```python
from build123d import *

# Parameters (mm, degrees)
BOSS_EXTRUDE1_START     = 7.2
SKETCH1_W               = 6
SKETCH1_H               = 3
BOSS_EXTRUDE1_DEPTH     = 24.3
BOSS_EXTRUDE2_START     = 28.5
SKETCH2_W               = 3
SKETCH2_H               = 35.475
BOSS_EXTRUDE2_DEPTH     = 21.5
CUT_EXTRUDE1_DEPTH      = 60.023009285
CUT_EXTRUDE1_DEPTH_BACK = 60.023009285
SKETCH3_R               = 1.2
SKETCH3_R_2             = 0.9
CUT_EXTRUDE2_DEPTH      = 60.023009285
CUT_EXTRUDE2_DEPTH_BACK = 60.023009285
SKETCH4_W               = 11
SKETCH4_H               = 1.2
SKETCH4_W_2             = 17
SKETCH4_H_2             = 12.475
CUT_EXTRUDE3_DEPTH      = 60.023009285
CUT_EXTRUDE3_DEPTH_BACK = 60.023009285
SKETCH5_W               = 3
SKETCH5_H               = 2.5


with BuildPart() as part:
    # Sketch1 → Boss-Extrude1 (new body)
    with BuildSketch(Plane.XY.offset(BOSS_EXTRUDE1_START)):
        with Locations((17.8, 21.975)):
            Rectangle(SKETCH1_W, SKETCH1_H)
    extrude(amount=BOSS_EXTRUDE1_DEPTH)

    # Sketch2 → Boss-Extrude2 (add)
    with BuildSketch(Plane.XY.offset(BOSS_EXTRUDE2_START)):
        with Locations((17.8, 5.7375)):
            Rectangle(SKETCH2_W, SKETCH2_H)
    extrude(amount=BOSS_EXTRUDE2_DEPTH)

    # Sketch3 → Cut-Extrude1 (cut, two sides: drawn at the far end of the back side and taken through both)
    with BuildSketch(Plane(origin=(0, 0, 0), x_dir=(1, 0, 0), z_dir=(0, 1, 0)).offset(-CUT_EXTRUDE1_DEPTH_BACK)):
        with Locations(Location((17.8, -24.5, 0), (0, 0, 270))):
            Circle(SKETCH3_R)
        with Locations(Location((17.8, -10.2, 0), (0, 0, 270))):
            Circle(SKETCH3_R_2)
    extrude(amount=CUT_EXTRUDE1_DEPTH + CUT_EXTRUDE1_DEPTH_BACK, mode=Mode.SUBTRACT)

    # Sketch4 → Cut-Extrude2 (cut, two sides: drawn at the far end of the back side and taken through both)
    with BuildSketch(Plane(origin=(0, 0, 0), x_dir=(0, 0, -1), z_dir=(1, 0, 0)).offset(-CUT_EXTRUDE2_DEPTH_BACK)):
        with Locations((-45.5, -6)):
            Rectangle(SKETCH4_W, SKETCH4_H)
        with Locations((-45.5, 0)):
            Rectangle(SKETCH4_W, SKETCH4_H)
        with Locations((-45.5, 6)):
            Rectangle(SKETCH4_W, SKETCH4_H)
        with Locations((-42.5, 18.2375)):
            Rectangle(SKETCH4_W_2, SKETCH4_H_2)
    extrude(amount=CUT_EXTRUDE2_DEPTH + CUT_EXTRUDE2_DEPTH_BACK, mode=Mode.SUBTRACT)

    # Sketch5 → Cut-Extrude3 (cut, two sides: drawn at the far end of the back side and taken through both)
    with BuildSketch(Plane(origin=(0, 0, 0), x_dir=(0, 0, -1), z_dir=(1, 0, 0)).offset(-CUT_EXTRUDE3_DEPTH_BACK)):
        with Locations((-49.5, -11.75)):
            Rectangle(SKETCH5_W, SKETCH5_H)
        with Locations((-49.5, 11.75)):
            Rectangle(SKETCH5_W, SKETCH5_H)
    extrude(amount=CUT_EXTRUDE3_DEPTH + CUT_EXTRUDE3_DEPTH_BACK, mode=Mode.SUBTRACT)


solid = part.part
```
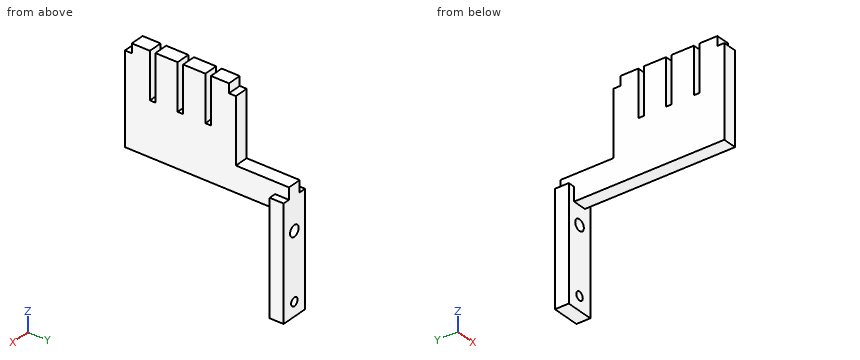
Verification items for the finished model (mm, model axes). Round coordinates to 2 decimals unless told otherwise and drop trailing zeros. Write each loop counter-clockwise with the first axis right and the second up, starting at its lowest first coordinate (ties: lowest second). Pieces come first, ordered by that corner, then holes.
1. Section check C-C on z = 10.2. Enter the section's corners in (x, y) (3 decimals), plus the area to 3 significant figures.
2. Scan lines: L1, parallel to Z at x = 17.8, y = 21.7; L2, parallel to Y at x = 19, z = 41.5; L3, parallel to X at y = 21.55, z = 24.5. Record each from-to range of solid material in increasing order.
3. Section check D-D on y = 15.5. Enter the section's corners in (x, z).
4. Section check B-B on z = 44. Enter the section's corners in (x, y), plus the area to 3 significant figures.
5. Gauge pin test, flat ends, axial feed: P1, Ø1, axis at x = 17.5, y = 6, coming from the +Z side; P2, Ø1.5, axis at x = 17.5, z = 46, coming from the +Y side; P3, Ø6.5, axis at y = 11, z = 38, coming from the +X side. Record the tip position at first contact, or that the pin passes through.
6. Section check A-A on x = 17.8. State how many separate pieces and enclosed holes the cut face has, plus the area to 3 significant figures.
Answer:
1. outline: (14.8, 20.475) - (16.9, 20.475) - (16.9, 23.475) - (14.8, 23.475) - close; (18.7, 20.475) - (20.8, 20.475) - (20.8, 23.475) - (18.7, 23.475) - close
1. area: 12.6 mm2
2. L1: z = 7.2 to 9.3, 11.1 to 23.3, 25.7 to 34
2. L2: y = -12 to -6.6, -5.4 to -0.6, 0.6 to 5.4, 6.6 to 12
2. L3: x = 14.8 to 16.6, 19 to 20.8
3. outline: (16.3, 28.5) - (19.3, 28.5) - (19.3, 34) - (16.3, 34) - close
4. outline: (16.3, -12) - (19.3, -12) - (19.3, -6.6) - (16.3, -6.6) - close; (16.3, -5.4) - (19.3, -5.4) - (19.3, -0.6) - (16.3, -0.6) - close; (16.3, 0.6) - (19.3, 0.6) - (19.3, 5.4) - (16.3, 5.4) - close; (16.3, 6.6) - (19.3, 6.6) - (19.3, 12) - (16.3, 12) - close
4. area: 61.2 mm2
5. P1: stops at z = 40
5. P2: stops at y = 12
5. P3: stops at x = 19.3
6. separate pieces: 3
6. enclosed holes: 0
6. area: 588 mm2
